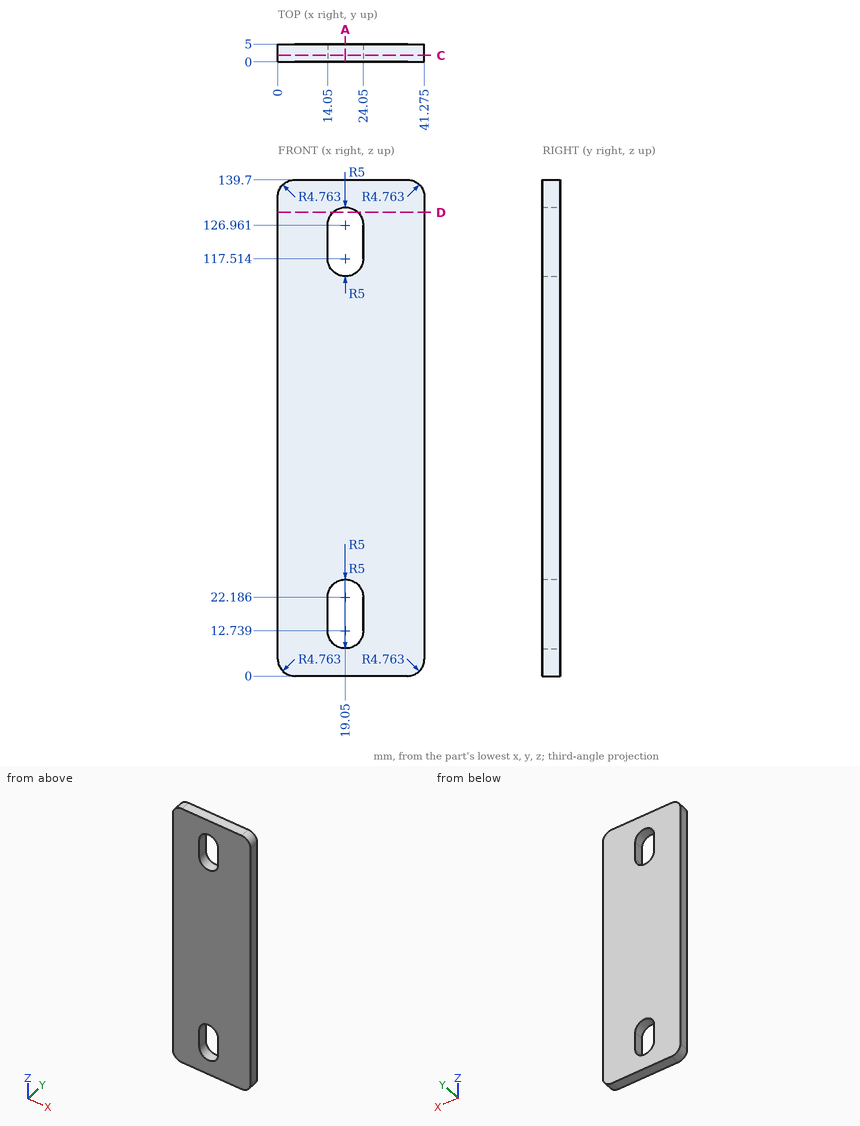
Here's the drawing with two shaded views (mm, measured from the low corner). I have some questions. Coordinates: 2 decimals unless noted, no trailing zeros. Loops run counter-clockwise (first coordinate to the right, second up) from the corner with the lowest first, then second, coordinate; pieces in that order, holes last. Notation, with made-up numbers: (43.5, -1.5) -> (52.5, -1.5) arc R23 ccw to (52.5, 14.5) -> close; hole circle Ø10 at (52, -26). An arc over 180 degrees is marked (long way). Put each result on its own line as item: value. Start each with the question number.
Q1. I want a section at A-A (x = 19.05). Write out the boundary of the cut face in (y, z) (1 decimal), plus the area to 3 significant figures.
Q2. If I drill on line 1 (Z direction, x = 15.5, y = 4.55) (1 decimal); line 2 (Z direction, x = 17, y = 1.55) (1 decimal); line 3 (X direction, y = 4.5, z = 131) (1 decimal), over which ranges is the centre line in solid material (lowest first)? Write a range as [from, to].
Q3. I want a section at D-D (z = 130.5). Write out the boundary of the cut face in (x, y) (1 decimal), plus the area to 3 significant figures.
Q4. I want a section at C-C (y = 1.8). Count the separate pieces of the cut face and the enclosed holes in it, plus the area to 3 significant figures.
Taken from the geometry:
1. outline: (0, 0) -> (5, 0) -> (5, 7.7) -> (0, 7.7) -> close; (0, 27.2) -> (5, 27.2) -> (5, 112.5) -> (0, 112.5) -> close; (0, 132) -> (5, 132) -> (5, 139.7) -> (0, 139.7) -> close
1. area: 504 mm2
2. line 1: z = [0, 9.2], [25.7, 114], [130.5, 139.7]
2. line 2: z = [0, 8.2], [26.7, 113], [131.5, 139.7]
2. line 3: x = [0, 16.1], [22, 41.3]
3. outline: (0, 0) -> (15.5, 0) -> (15.5, 5) -> (0, 5) -> close; (22.6, 0) -> (41.3, 0) -> (41.3, 5) -> (22.6, 5) -> close
3. area: 171 mm2
4. separate pieces: 1
4. enclosed holes: 2
4. area: 5,400 mm2
